Autodesk Inventor part; units mm, degrees
ref_plane "Work Plane1" through (1.525, 0, 0) normal (0, 0, 1) x (1, 0, 0)
ref_plane "YZ Plane" through (0, 0, 0) normal (1, 0, 0) x (0, 1, 0)
ref_plane "XZ Plane" through (0, 0, 0) normal (0, 1, 0) x (-1, 0, 0)
sketch "Sketch1" plane through (0, 0, 0) normal (0, 0, 1) x (1, 0, 0)
  line L0 (0, 5.5626) -> (0, 3.302)
  line L1 (38.1, 3.175) -> (57.15, 3.175)
  line L2 (57.15, 3.175) -> (57.15, 0)
  line L3 (57.15, 0) -> (-0.0001, 0)
  line L4 (-11.4301, 0) -> (68.58, 0)
  line L5 (-0.0001, 0) -> (-0.0001, 5.5626)
  line L6 (-0.0001, 5.5626) -> (0, 5.5626)
  line L7 (38.1, 3.175) -> (34.9249, 3.302)
  line L8 (34.9249, 3.302) -> (0, 3.302)
  line L9 (0, -1.1125) -> (0, 6.6751)
  dimension "d0" = 57.15
  dimension "d1" = 19.05
  dimension "d2" = 6.35
  dimension "d9" = 0.0001
  dimension "d10" = 11.1252
  dimension "d13" = 3.1751
  dimension "d14" = 6.604
revolve "Body" add sketch "Sketch1" angle 360 about axis through (57.15, 0, 0) along (-1, 0, 0)
sketch "Sketch2" plane through (-0.0001, 0, 0) normal (-1, 0, 0) x (0, 0, 1)
  line L0 (0, 6.4231) -> (5.5626, 3.2116)
  line L1 (5.5626, 3.2116) -> (5.5626, -3.2116)
  line L2 (5.5626, -3.2116) -> (0, -6.4231)
  line L3 (0, -6.4231) -> (-5.5626, -3.2116)
  line L4 (-5.5626, -3.2116) -> (-5.5626, 3.2116)
  line L5 (-5.5626, 3.2116) -> (0, 6.4231)
  point P0 (0, 0)
  point P1 (0, 0)
  dimension "d11" = 11.1252
extrude "Head" add sketch "Sketch2" along normal blind 4.7752
sketch "Sketch4" plane through (0, 0, 0) normal (0, 0, 1) x (1, 0, 0)
  line L0 (-4.7753, 5.5626) -> (-4.7753, 6.4231)
  line L1 (-4.7753, 6.4231) -> (-4.2785, 6.4231)
  line L2 (-4.2785, 6.4231) -> (-4.7753, 5.5626)
  line L3 (-5.7303, 0) -> (0.9549, 0)
  line L4 (-0.0001, 6.4231) -> (-4.7753, 6.4231)
  line L5 (-4.7753, 3.2116) -> (-4.7753, 6.4231)
  dimension "d5" = 30
  dimension "d19" = 11.1252
revolve "Chamfer1" cut sketch "Sketch4" angle 360 about axis through (-10, 0, 0) along (1, 0, 0)
thread "Thread"
chamfer "Chamfer2" distance 0.7791 distance2 0.7557 1 edges at (57.15, -3.175, 0) measured on face at (57.15, -1.44, -0.4308)
ref_plane "Work Plane1" through (1.525, 0, 0) normal (0, 0, 1) x (1, 0, 0)
fillet "Fillet2" radius 0.762 1 edges at (0, -3.302, 0)
equation "\"d0\" = NLG"
equation "\"d1\" = GEL"
equation "\"d2\" = GD"
equation "\"d10\" = SD2"
equation "\"d14\" = BDM"
equation "\"d11\" = SW"
equation "\"d3\" = KOH - SD"
equation "\"d5\" = ANG1"
equation "\"d19\" = SW0"
equation "\"d63\" = R"
equation "\"d15\" = GEL"
equation "\"d6\" = -0.5 * SPD + 0.5 * GD"
equation "\"NLG\" = 57.15"
equation "\"GD\" = NND"
equation "\"BDM\" = 6.604"
equation "\"KOH\" = 4.7752"
equation "\"GEL\" = 19.05"
equation "\"SW\" = 11.1252"
equation "\"SW0\" = SW"
equation "\"SPD\" = GD1"
equation "\"SD2\" = SW"
equation "\"SD\" = 0"
equation "\"ANG1\" = 30deg"
equation "\"GAL\" = 3.175"
equation "\"GUL\" = 0.238 * GAL"
equation "\"R\" = 0.762"
equation "\"d62\" = -NLG - SD + GUL"
equation "\"GD1\" = 4.79184"
equation "\"THREADDIA\" = 6.35"
equation "\"TOA\" = 30deg"
equation "\"NND\" = 6.35"
equation "\"E0\" = 1.155 * SW"
properties part number "ANSI/ASME B18.2.1 - 1/4-20 UNC - 2.25" material "Steel, Mild"
Geometry: final body of the model. Coordinates: model frame, mm. A direction names the side the tool comes from. Give positions to 0.01 mm unless a question says otherwise; leave off trailing zeros. Write each loop counter-clockwise with the first axis right and the second up, starting at its lowest first coordinate (ties: lowest second). Pieces come first, ordered by that corner, then holes. Notation, with made-up numbers: (-35, -34) -> (-17, -34) arc R25 ccw to (-17, 4) -> close; hole circle Ø3 at (29, 34). An arc over 180 degrees is marked (long way). Answer as a JSON object with one key per item and string values.
1. Ray query, probe 1 along Y at (x, z) = (38, 0); probe 2 along X at (y, z) = (2.25, 3.75); probe 3 along Z at (x, y) = (20.5, -0.25). Return the intervals inside material, ascending. Write a range as from..to.
Ans:
{"probe 1": "y = -3.18..3.18", "probe 2": "x = -4.78..0", "probe 3": "z = -3.29..3.29"}
2. Contact query for flat-ended pins moving along their axis: pin 1 (2 mm diameter, centred on x = 28.5, y = 3, fed in from -Z); pin 2 (5 mm diameter, centred on x = 5.5, z = 1, fed in from +Y); pin 3 (4 mm diameter, centred on x = 10, z = -4.5, fed in from -Y). Output: stop coordinate, or through.
Ans:
{"pin 1": "stops at z = -2.63", "pin 2": "stops at y = 3.3", "pin 3": "stops at y = -2.16"}
3. Cut plane B-B on x = 47. Output: boundary loops of the cut face in (y, z) (3 decimals).
Ans:
{"outline": "circle Ø6.35 at (0, 0)"}
4. Access query for faces 1 (the cylindrical face through (47.38, -0.69, -3.1)), 2 (the flat face through (-2, 0, -5.563)). Directions: +Z, -Z, +X, -X, +Y, -Y. A direction counts if a zero-diameter tool reaches every point of the face in a straight line with its end or side. Return the directions, or none.
Ans:
{"face 1": "+X", "face 2": "-Z, +X, -X, +Y, -Y"}
5. Cut plane A-A on x = 26.5. Output: boundary loops of the cut face in (y, z).
Ans:
{"outline": "circle Ø6.6 at (0, 0)"}
